Read the model definition and answer for the solid it produces. Units are mm, in the model's axes. Give positions to 0.01 mm unless a question says otherwise; leave off trailing zeros. Order: outer loops, then holes, each group sorted by start corner. A loop starts at its lowest first (then second) coordinate and runs counter-clockwise, first axis right, second up. Notation, with made-up numbers: (14.5, -11.75) - (55.5, -11.75) arc R29 ccw to (55.5, 18.25) - close; hole circle Ø6 at (-33, 75). An arc over 180 degrees is marked (long way). Use a Markdown table: item, result. Add a question column.
1. For a pull along Z with two mould halves and no side action, classify faces 1 (the flat face through (0, 4, -180.732)), 2 (the flat face through (4, 4, -249)), 3 (the cylindrical face through (0.325, 3.944, -318.463)) as released by +Z, released by -Z, zero draft, split by the parting line, or undercut.
2. A flat-ended cylindrical pin translates along its axis: P1, Ø1.8, axis at x = 0, z = -319.927, coming from the +Y side. Find the tip coordinate at first contact, or state that the pin passes through.
3. A cutting plane is placed at A-A on x = 0. Determine the outline of the cut face in (y, z).
4. Consider L1, parallel to Z at x = 0, y = 6; L2, parallel to Z at x = 0.5, y = 4; L3, parallel to Z at x = -2.25, y = 4.5. Determine where each line is inside the solid, lowest interval first.
Autodesk Inventor part; units mm, degrees
ref_plane "XZ Plane" through (0, 0, 0) normal (0, 1, 0) x (-1, 0, 0)
ref_plane "XY Plane" through (0, 0, 0) normal (0, 0, 1) x (1, 0, 0)
sketch "Sketch1" plane through (0, 0, 0) normal (0, 1, 0) x (-1, 0, 0)
  line L0 (0, 0) -> (0, -319.927) construction
  line L1 (-4, 0) -> (-4, -319.927)
  line L2 (4, -319.927) -> (4, 0)
  arc A0 (4, 0) -> (-4, 0) centre (0, 0) ccw
  arc A1 (-4, -319.927) -> (4, -319.927) centre (0, -319.927) ccw
  circle A2 centre (0, 0) radius 1.5
  circle A3 centre (0, -319.927) radius 1.5
  line L3 (0, -50.8) -> (0, -100) construction
  line L4 (-1.5, -50.8) -> (-1.5, -100)
  line L5 (1.5, -100) -> (1.5, -50.8)
  arc A4 (1.5, -50.8) -> (-1.5, -50.8) centre (0, -50.8) ccw
  arc A5 (-1.5, -100) -> (1.5, -100) centre (0, -100) ccw
  arc A6 (4, 0) -> (4, -40) centre (202.9975, -20) ccw
  arc A7 (-4, 0) -> (-4, -40) centre (194.9975, -20) ccw
  point P0 (0, -159.9635)
  point P1 (0, -75.4)
  dimension "d0" = 319.927
  dimension "d1" = 8
  dimension "d2" = 3
  dimension "d3" = 3
  dimension "d12" = 3
  dimension "d13" = 50.8
  dimension "d14" = 100
  dimension "d15" = 40
  dimension "d16" = 200
  dimension "d17" = 200
extrude "Extrusion1" add sketch "Sketch1" along normal blind 8 contours A0 A6 L2 A1 L1 | L1 A7
sketch "Sketch2" plane through (0, 0, 0) normal (0, -1, 0) x (1, 0, 0)
  arc A0 (4, -40) -> (4, 0) centre (-194.9975, -20) ccw
  arc A1 (4, 0) -> (-4, 0) centre (0, 0) ccw
  arc A2 (-4, -40) -> (-4, 0) centre (-202.9975, -20) ccw
  line L0 (-4, -319.927) -> (-4, -40)
  arc A3 (-4, -319.927) -> (4, -319.927) centre (0, -319.927) ccw
  line L1 (4, -40) -> (4, -319.927)
  circle A4 centre (0, 0) radius 1.5
  circle A5 centre (0, -319.927) radius 1.5
  arc A6 (1.5, -50.8) -> (-1.5, -50.8) centre (0, -50.8) ccw
  line L2 (1.5, -100) -> (1.5, -50.8)
  arc A7 (-1.5, -100) -> (1.5, -100) centre (0, -100) ccw
  line L3 (-1.5, -50.8) -> (-1.5, -100)
sketch "Sketch3" plane through (0, 8, 0) normal (0, 1, 0) x (1, 0, 0)
  line L0 (-21.634, 180.7321) -> (39.8396, 180.7321)
  line L1 (39.8396, 180.7321) -> (39.8396, -20.7362)
  line L2 (39.8396, -20.7362) -> (-21.634, -20.7362)
  line L3 (-21.634, -20.7362) -> (-21.634, 180.7321)
  line L4 (-50.5628, 342.9399) -> (62.0528, 342.9399)
  line L5 (62.0528, 342.9399) -> (62.0528, -55.3474)
  line L6 (62.0528, -55.3474) -> (-50.5628, -55.3474)
  line L7 (-50.5628, -55.3474) -> (-50.5628, 342.9399)
  point P0 (0, 0)
extrude "Extrusion2" cut sketch "Sketch3" along normal mid plane 20 contours L0 L1 L2 L3
sketch "Sketch4" plane through (0, 8, 0) normal (0, 1, 0) x (1, 0, 0)
  line L0 (-4, 180.7321) -> (4, 180.7321)
  line L1 (-4, 319.927) -> (-4, 180.7321)
  line L2 (4, 180.7321) -> (4, 319.927)
  arc A0 (4, 319.927) -> (-4, 319.927) centre (0, 319.927) ccw
  point P0 (0, 0)
properties part number "Part_8_p2"
Output values:
| question | item | result |
|---|---|---|
| 1 | face 1 | released by +Z |
| 1 | face 2 | zero draft |
| 1 | face 3 | undercut |
| 2 | P1 | through |
| 3 | outline | (0, -323.93) - (8, -323.93) - (8, -321.43) - (0, -321.43) - close; (0, -318.43) - (8, -318.43) - (8, -180.73) - (0, -180.73) - close |
| 4 | L1 | -323.93 to -321.43, -318.43 to -180.73 |
| 4 | L2 | -323.9 to -321.34, -318.51 to -180.73 |
| 4 | L3 | -323.23 to -180.73 |
